Could you check a few things on this model? Use its own coordinates, in mm. Coordinates: 2 decimals unless noted, no trailing zeros. Write each loop counter-clockwise with the first axis right and the second up, starting at its lowest first coordinate (ties: lowest second). Pieces come first, ordered by that corner, then holes. Notation, with made-up numbers: M -18,29 L 30,29 A24 ccw 30,62 Z; hole C 81,-15 d10. An arc over 180 degrees is marked long. Write item = value, one per line.
```python
from build123d import *

# Parameters (mm, degrees)
SKETCH_1_R          = 1.5
SKETCH_1_R_2        = 8
SKETCH_1_R_3        = 1.1
SKETCH_1_R_4        = 10.5
EXTRUDE_1_DEPTH     = 4
SKETCH_3_W          = 30
SKETCH_3_H          = 6
CUT_EXTRUDE_1_DEPTH = 5
FILLET_4_R          = 3
CHAMFER_1_SIZE      = 25
FILLET_8_R          = 5
FILLET_12_R         = 2
FILLET_13_R         = 3
FILLET_14_R         = 10


with BuildPart() as part:
    # 草图1 → 凸台-拉伸1 (new body)
    with BuildSketch(Plane(origin=(0, 0, 0), x_dir=(1, 0, 0), z_dir=(0, 1, 0))):
        Polygon((-20, 17.5), (-20, -97.5), (23, -97.5), (23, 17.5), (23, 87.5), (33, 87.5), (33, 97.5), (-33, 97.5), (-33, 87.5), (-20, 87.5), align=None)
        with Locations(Location((-10, -93.5, 0), (0, 0, 270))):
            Circle(SKETCH_1_R, mode=Mode.SUBTRACT)
        with Locations(Location((-2, -65.5, 0), (0, 0, 270))):
            Circle(SKETCH_1_R_2, mode=Mode.SUBTRACT)
        with Locations(Location((-10, -45.5, 0), (0, 0, 270))):
            Circle(SKETCH_1_R, mode=Mode.SUBTRACT)
        with Locations(Location((10, -71.5, 0), (0, 0, 270))):
            Circle(SKETCH_1_R, mode=Mode.SUBTRACT)
        with Locations(Location((10, -45.5, 0), (0, 0, 270))):
            Circle(SKETCH_1_R, mode=Mode.SUBTRACT)
        Polygon((-10, 0), (10, 0), (13, 0), (13, -30), (10, -30), (-10, -30), align=None, mode=Mode.SUBTRACT)
        with Locations(Location((-27.5, 95, 0), (0, 0, 270))):
            Circle(SKETCH_1_R_3, mode=Mode.SUBTRACT)
        with Locations(Location((-1, 76, 0), (0, 0, 270))):
            Circle(SKETCH_1_R_4, mode=Mode.SUBTRACT)
        with Locations(Location((22.3, 90.5, 0), (0, 0, 270))):
            Circle(SKETCH_1_R_3, mode=Mode.SUBTRACT)
        with Locations(Location((22.3, 94.5, 0), (0, 0, 270))):
            Circle(SKETCH_1_R_3, mode=Mode.SUBTRACT)
    extrude(amount=EXTRUDE_1_DEPTH)

    # 草图3 → 切除-拉伸1 (cut)
    with BuildSketch(Plane(origin=(0, 4, 0), x_dir=(1, 0, 0), z_dir=(0, 1, 0))):
        with Locations((0, 94.5)):
            Rectangle(SKETCH_3_W, SKETCH_3_H)
    extrude(amount=-CUT_EXTRUDE_1_DEPTH, mode=Mode.SUBTRACT)

    # 圆角4
    fillet_4_edges = [part.edges().sort_by_distance(p)[0] for p in [
        (15, 2, -91.5),
        (-15, 2, -91.5),
    ]]
    fillet(fillet_4_edges, radius=FILLET_4_R)
    fillet_4_2_edges = [part.edges().sort_by_distance(p)[0] for p in [
        (15, 2, -97.5),
        (-15, 2, -97.5),
    ]]
    fillet(fillet_4_2_edges, radius=FILLET_4_R - 0.0001)  # a hair under: the kernel refuses the full size

    # 倒角1
    chamfer_1_edges = [part.edges().sort_by_distance(p)[0] for p in [
        (23, 2, 97.5),
    ]]
    chamfer(chamfer_1_edges, length=CHAMFER_1_SIZE)

    # 圆角8
    fillet_8_edges = [part.edges().sort_by_distance(p)[0] for p in [
        (13, 2, 0),
        (-10, 2, 0),
        (-10, 2, 30),
        (13, 2, 30),
    ]]
    fillet(fillet_8_edges, radius=FILLET_8_R)

    # 圆角12
    fillet_12_edges = [part.edges().sort_by_distance(p)[0] for p in [
        (-33, 2, -87.5),
        (-33, 2, -97.5),
        (33, 2, -97.5),
        (33, 2, -87.5),
    ]]
    fillet(fillet_12_edges, radius=FILLET_12_R)

    # 圆角13
    fillet_13_edges = [part.edges().sort_by_distance(p)[0] for p in [
        (23, 2, 72.5),
        (-2, 2, 97.5),
        (-20, 2, 97.5),
    ]]
    fillet(fillet_13_edges, radius=FILLET_13_R)

    # 圆角14
    fillet_14_edges = [part.edges().sort_by_distance(p)[0] for p in [
        (23, 2, -87.5),
        (-20, 2, -87.5),
    ]]
    fillet(fillet_14_edges, radius=FILLET_14_R)


solid = part.part
```
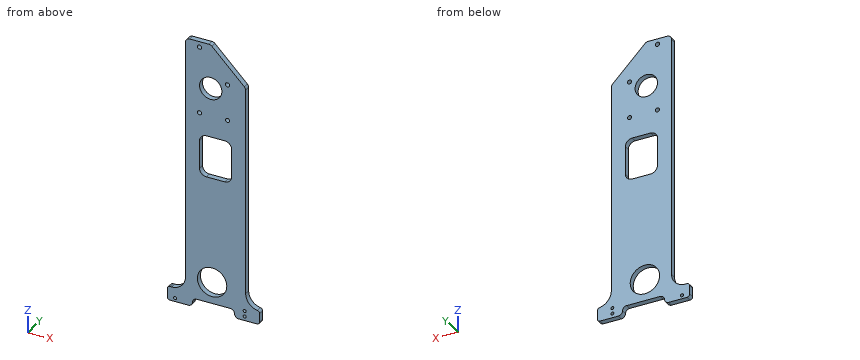
Item 1: Imagine slicing it at C-C (y = 3). State how many separate pieces and enclosed holes the cut face has, and give its area (3 significant figures).
Numbers:
separate_pieces = 1
enclosed_holes = 10
area = 6,900 mm²
Item 2: Imagine slicing it at D-D (z = -63.5). Write out the boundary of the cut face in (x, y).
Numbers:
outline = M -20,0 L 23,0 L 23,4 L -20,4 Z
Item 3: Imagine slicing it at B-B (z = 65.5). Write out the boundary of the cut face in (x, y).
Numbers:
outline = M -20,0 L -10,0 L -10,4 L -20,4 Z; M 6,0 L 23,0 L 23,4 L 6,4 Z
Item 4: Imagine slicing it at A-A (z = 2). Write out the boundary of the cut face in (x, y), and give its area (3 significant figures).
Numbers:
outline = M -20,0 L -9,0 L -9,4 L -20,4 Z; M 12,0 L 23,0 L 23,4 L 12,4 Z
area = 88.0 mm²
Item 5: If I drill on line 1 along Z through (x, y) = (22, 1.3); line 2 along X through (y, z) = (0.9, -94.5); line 3 along Z through (x, y) = (0, 3.7), over which ranges is the centre line in solid material (lowest first)?
Numbers:
line_1 = -97.5 to -95.56, -93.44 to -91.56, -89.44 to 73.5
line_2 = -33 to -28.48, -26.52 to -15, 15 to 21.2, 23.4 to 33
line_3 = -91.5 to -86.45, -65.55 to 0, 30 to 57.75, 73.25 to 95.5
Item 6: I'm going to push flat-ended pins straight in: P1, Ø1.5, axis at x = 13, y = 3.5, coming from the -Z side; P2, Ø2, axis at x = 3.5, y = 2, coming from the -Z side; P3, Ø1.5, axis at y = 2, z = -39, coming from the +X side; P4, Ø1.3, axis at x = 22.3, z = -90.5, coming from the -Y side. Where does each tip first touch, or does it pass through?
Numbers:
P1 = -92.06
P2 = -91.5
P3 = 23
P4 = through
